Autodesk Fusion 360 part; units mm, degrees
sketch "Sketch1" plane through (0, 0, 0) normal (0, 1, 0) x (1, 0, 0)
  circle A0 centre (0, 0) radius 10
  line L0 (0, 40) -> (80, 40)
  line L1 (20, 0) -> (20, 25)
  line L2 (20, 25) -> (80, 25)
  arc A1 (0, 20) -> (20, 0) centre (0, 0) ccw
  line L3 (80, 25) -> (90, 25)
  line L4 (90, 25) -> (90, 45)
  line L5 (90, 45) -> (80, 45)
  line L6 (80, 45) -> (80, 40)
  line L7 (0, 20) -> (0, 40)
  dimension "d1" = 20
  dimension "d2" = 40
  dimension "d3" = 40
  dimension "d4" = 80
  dimension "d5" = 15
  dimension "d6" = 5
  dimension "d7" = 10
extrude "Extrude1" add sketch "Sketch1" along normal mid plane 40
sketch "Sketch2" plane through (0, 0, 0) normal (0, 1, 0) x (1, 0, 0)
sketch "Sketch3" plane through (0, 0, -25) normal (0, 0, 1) x (-1, 0, 0)
  line L0 (-90, 20) -> (-90, -20)
  line L1 (-90, -20) -> (-20, -20)
  line L2 (-20, -20) -> (-20, 20)
  line L3 (-20, 20) -> (-90, 20)
  circle A0 centre (-65, 0) radius 7.5
  dimension "d10" = 15
  dimension "d11" = 25
  dimension "d12" = 20
extrude "Extrude2" cut sketch "Sketch3" against normal blind 40 contours A0
ref_plane "WorkPlane1" through (35, 0, -12.5) normal (0, -1, 0) x (-1, 0, 0)
sketch "Sketch4" plane through (0, 0, 0) normal (0, -1, 0) x (-1, 0, 0)
  line L0 (-20, 0) -> (-40, 25)
  line L1 (-20, 0) -> (-20, 25)
  line L2 (-20, 25) -> (-40, 25)
extrude "Extrude3" add sketch "Sketch4" along normal mid plane 10
Design review of the part built by this model. Coordinates are the model's own, in mm. A direction names the side the tool comes from. Round coordinates to 2 decimals unless told otherwise and drop trailing zeros. Loops run counter-clockwise (first coordinate to the right, second up) from the corner with the lowest first, then second, coordinate; pieces in that order, holes last. Notation, with made-up numbers: (19, -32.75) - (29, -32.75) arc R19 ccw to (29, -25.75) - close; hole circle Ø1 at (86.5, 17). An arc over 180 degrees is marked (long way). One line per item, written item: value. Start each with the question number.
1) Draft analysis for pull direction X (two halves, no side actions). For faces 1 (the cylindrical face through (72.493, -0.33, -32.395)), 2 (the flat face through (80, 0, -43)), 3 (the flat face through (20, 12, -12)), state which applies: +X half, -X half, draft (parallel to the pull), parting line (faces both ways), or undercut.
2) Consider section A-A on y = 0. Give the boundary of the cut face in (x, z).
3) Consider section D-D on x = 24. Give the boundary of the cut face in (y, z).
4) To check wall thickness, follow L1, parallel to X at y = 8.5, z = 0; L2, parallel to Z at x = 5.5, y = -11.5; L3, parallel to Z at x = 78, y = 7.5. State the ranges of each line that lie inside material, in increasing order. Write a range as from..to.
5) Consider section B-B on x = 65. Give the boundary of the cut face in (y, z), then the cut area to 3 significant figures.
6) Insertion check: pin 1 Ø3 at (x, y) = (10, -3.5) entering from +Z; pin 2 Ø19.5 at (x, y) = (65, 0) entering from +Z; pin 3 Ø10 at (x, y) = (21.5, 4.5) entering from +Z. Each pin has a flat end and moves straight along its axis. Give the tip position at first contact, or say it passes through.
7) For faces 4 (the flat face through (55, 0, -25)), 5 (the flat face through (0, 0, -30)), 6 (the flat face through (26, -5, -18)), 7 (the flat face through (26, 5, -18)), list the 3-axis set-ups (+Z, -Z, +X, -X, +Y, -Y) from which the entire face can be reached by the end or side of a thin tool; tool diameter is ignored.
8) Consider section C-C on y = -9. Give the boundary of the cut face in (x, z).
Reported:
1. face 1: undercut
1. face 2: -X half
1. face 3: +X half
2. outline: (0, -40) - (57.5, -40) - (57.5, -25) - (40, -25) - (20, 0) arc R20 ccw (long way) to (0, -20) - close; (72.5, -40) - (80, -40) - (80, -45) - (90, -45) - (90, -25) - (72.5, -25) - close; hole circle Ø20 at (0, 0)
3. outline: (-20, -40) - (20, -40) - (20, -25) - (5, -25) - (5, -5) - (-5, -5) - (-5, -25) - (-20, -25) - close
4. L1: x = -20..-10, 10..20
4. L2: z = -40..-8.35, 8.35..19.23
4. L3: z = -40..-25
5. outline: (-20, -40) - (-7.5, -40) - (-7.5, -25) - (-20, -25) - close; (7.5, -40) - (20, -40) - (20, -25) - (7.5, -25) - close
5. area: 375 mm^2
6. pin 1: stops at z = 18.1
6. pin 2: stops at z = -25
6. pin 3: stops at z = 11.3
7. face 4: +Z, +X
7. face 5: -Z, -X, +Y, -Y
7. face 6: +Z, +X, -Y
7. face 7: +Z, +X, +Y
8. outline: (0, -40) - (80, -40) - (80, -45) - (90, -45) - (90, -25) - (20, -25) - (20, 0) arc R20 ccw (long way) to (0, -20) - close; hole circle Ø20 at (0, 0)
